The listing builds one solid part. Answer for the finished solid, in the listing's coordinates (mm). Round coordinates to 2 decimals unless told otherwise and drop trailing zeros. Write each loop counter-clockwise with the first axis right and the second up, starting at its lowest first coordinate (ties: lowest second). Pieces come first, ordered by that corner, then holes. Notation, with made-up numbers: M 66.25,85 L 82.25,85 A28 cw 82.25,124 Z; hole C 25.5,41 d5. An arc over 180 degrees is marked long. One line per item, written item: value. Start each with the question number.
(1) Section B-B (z = 19.5) is taken. Determine the outline of the cut face in (x, y), plus the area to 3 significant figures.
(2) Consider probe 1 along Y at (x, z) = (8, 21.5); probe 2 along Y at (x, z) = (21, 4.25); probe 3 along X at (y, z) = (24.5, 15.75). Determine where each line is inside the solid, lowest interval first.
(3) Section D-D (y = 13.5) is taken. Determine the outline of the cut face in (x, z), plus the area to 3 significant figures.
(4) Section A-A (x = 19) is taken. Determine the outline of the cut face in (y, z).
```python
from build123d import *

# Parameters (mm, degrees)
F1_DEPTH = 25.4


with BuildPart() as f1:
    # F0 (on Top) → F1 (new body)
    with BuildSketch(Plane.XY):
        with BuildLine():
            ThreePointArc((0, 28.596171), (20.220547, 20.220547), (28.596171, 0))
            ThreePointArc((28.596171, 0), (20.220547, -20.220547), (0, -28.596171))
            Line((0, -28.596171), (53.911736, -28.596171))
            Line((53.911736, -28.596171), (53.911736, 28.596171))
            Line((53.911736, 28.596171), (0, 28.596171))
        make_face()
    extrude(amount=F1_DEPTH)


solid = f1.part
```
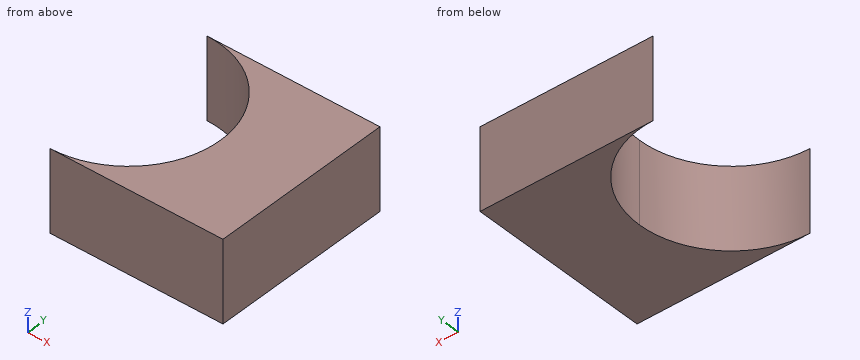
Recorded:
1. outline: M 0,-28.6 L 53.91,-28.6 L 53.91,28.6 L 0,28.6 A28.6 cw 28.6,0 A28.6 cw Z
1. area: 1,800 mm2
2. probe 1: y = -28.6 to -27.45, 27.45 to 28.6
2. probe 2: y = -28.6 to -19.41, 19.41 to 28.6
2. probe 3: x = 14.75 to 53.91
3. outline: M 25.21,0 L 53.91,0 L 53.91,25.4 L 25.21,25.4 Z
3. area: 729 mm2
4. outline: M -28.6,0 L -21.37,0 L -21.37,25.4 L -28.6,25.4 Z; M 21.37,0 L 28.6,0 L 28.6,25.4 L 21.37,25.4 Z
